The listing builds one solid part. Answer for the finished solid, in the listing's coordinates (mm). Face numbers are marked on the shaded views. A direction names the side the tool comes from. Give positions to 0.01 mm unless a question says otherwise; leave off trailing zeros. Loops run counter-clockwise (first coordinate to the right, second up) from the corner with the lowest first, then second, coordinate; pieces in that order, holes last. Notation, with made-up numbers: (-10.75, 79.5) - (44.25, 79.5) arc R25 ccw to (44.25, 106.5) - close; hole circle Ø2 at (-3, 63.5). An arc over 180 degrees is marked (long way). Write item = value, one per line. Start each with the question number.
1) The part is cut by section B-B on y = -2. Write down the section's boundary in (x, z).
2) The part is cut by section A-A on z = 44. Write down the section's boundary in (x, y), plus the area to 3 significant figures.
3) Flat-ended cylindrical pins translate along their axes: P1, Ø6, axis at x = 23, y = 14, coming from the -Z side; P2, Ø5, axis at x = 7, y = -21.5, coming from the +Z side. Find the tip coordinate at first contact, or state that the pin passes through.
4) Consider probe 1 along X at (y, z) = (20, 7.5); probe 2 along Z at (x, y) = (-4.5, -26). Determine where each line is inside the solid, lowest interval first.
5) Which of the six approach directions +Z, -Z, +X, -X, +Y, -Y give full straight-line access (tool end or side, diameter ignored) to the marked faces 1 and 2?
6) The mould has two halves that part along Y. Classify the marked faces 3, 4 and 5: +Y half, -Y half, draft (parallel to the pull), parting line (faces both ways), or undercut.
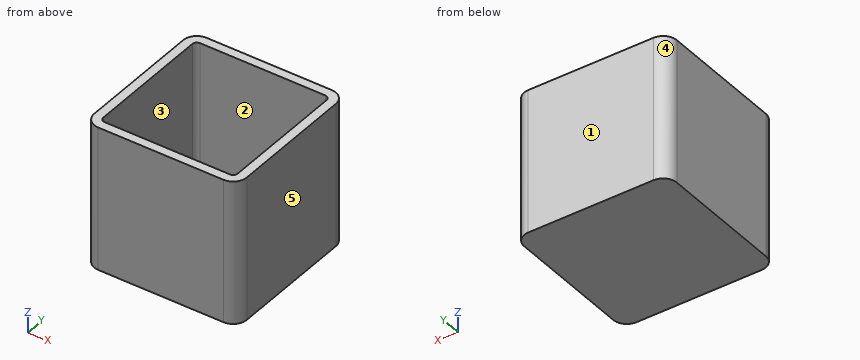
from build123d import *

# Parameters (mm, degrees)
F0_W     = 67
F0_H     = 67
F0_W_2   = 59
F0_H_2   = 59
F1_DEPTH = 4
F2_DEPTH = 63
F3_R     = 2
F4_R     = 6


with BuildPart() as f1:
    # F0 (on Top) → F1 (new body)
    with BuildSketch(Plane.XY):
        Rectangle(F0_W, F0_H)
        Rectangle(F0_W_2, F0_H_2, mode=Mode.SUBTRACT)
        Rectangle(F0_W_2, F0_H_2)
    extrude(amount=F1_DEPTH)

    # F0 (on Top) → F2 (join)
    with BuildSketch(Plane.XY):
        Rectangle(F0_W, F0_H)
        Rectangle(F0_W_2, F0_H_2, mode=Mode.SUBTRACT)
    extrude(amount=F2_DEPTH)

    # F3
    f3_edges = [f1.edges().sort_by_distance(p)[0] for p in [
        (29.5, -29.5, 33.5),
        (-29.5, -29.5, 33.5),
        (-29.5, 29.5, 33.5),
        (29.5, 29.5, 33.5),
        (-29.5, 0, 4),
        (0, 29.5, 4),
        (29.5, 0, 4),
        (0, -29.5, 4),
    ]]
    fillet(f3_edges, radius=F3_R)

    # F4
    f4_edges = [f1.edges().sort_by_distance(p)[0] for p in [
        (-33.5, 33.5, 31.5),
        (-33.5, -33.5, 31.5),
        (33.5, -33.5, 31.5),
        (33.5, 33.5, 31.5),
    ]]
    fillet(f4_edges, radius=F4_R)


solid = f1.part
Answer below:
q1.outline = (-33.5, 0) - (33.5, 0) - (33.5, 63) - (29.5, 63) - (29.5, 6) arc R2 cw to (27.5, 4) - (-27.5, 4) arc R2 cw to (-29.5, 6) - (-29.5, 63) - (-33.5, 63) - close
q2.outline = (-33.5, -27.5) arc R6 ccw to (-27.5, -33.5) - (27.5, -33.5) arc R6 ccw to (33.5, -27.5) - (33.5, 27.5) arc R6 ccw to (27.5, 33.5) - (-27.5, 33.5) arc R6 ccw to (-33.5, 27.5) - close; hole (-29.5, -27.5) arc R2 ccw to (-27.5, -29.5) - (27.5, -29.5) arc R2 ccw to (29.5, -27.5) - (29.5, 27.5) arc R2 ccw to (27.5, 29.5) - (-27.5, 29.5) arc R2 ccw to (-29.5, 27.5) - close
q2.area = 981 mm2
q3.P1 = 0
q3.P2 = 4
q4.probe_1 = -33.5 to -29.5, 29.5 to 33.5
q4.probe_2 = 0 to 4
q5.face_1 = +Z, -Z, +X, -X, +Y
q5.face_2 = +Z
q6.face_3 = undercut
q6.face_4 = +Y half
q6.face_5 = draft
